```python
from build123d import *

# Parameters (mm, degrees)
SKETCH1_R           = 60.625
SKETCH1_R_2         = 45
BOSS_EXTRUDE1_DEPTH = 4
SKETCH2_R           = 49
SKETCH2_R_2         = 45
BOSS_EXTRUDE2_DEPTH = 52
SKETCH3_W           = 8
SKETCH3_H           = 38
SKETCH3_W_2         = 15
SKETCH3_H_2         = 8
BOSS_EXTRUDE3_DEPTH = 13
SKETCH4_W           = 10
SKETCH4_H           = 24
CUT_EXTRUDE1_DEPTH  = 8
SKETCH5_R           = 5
CUT_EXTRUDE2_DEPTH  = 110.441337026
SKETCH6_R           = 1.3
CUT_EXTRUDE3_DEPTH  = 7.2
BOSS_EXTRUDE4_DEPTH = 4
SKETCH8_R           = 1.5
CUT_EXTRUDE4_DEPTH  = 103.404986506
FILLET1_R           = 1


with BuildPart() as part:
    # Sketch1 → Boss-Extrude1 (new body)
    with BuildSketch(Plane(origin=(0, 0, 0), x_dir=(1, 0, 0), z_dir=(0, 1, 0))):
        with Locations(Location((0, 0, 0), (0, 0, 270))):
            Circle(SKETCH1_R)
        with Locations(Location((0, 0, 0), (0, 0, 270))):
            Circle(SKETCH1_R_2, mode=Mode.SUBTRACT)
    extrude(amount=BOSS_EXTRUDE1_DEPTH)

    # Sketch2 → Boss-Extrude2 (add)
    with BuildSketch(Plane(origin=(0, 4, 0), x_dir=(1, 0, 0), z_dir=(0, 1, 0))):
        with Locations(Location((0, 0, 0), (0, 0, 90))):
            Circle(SKETCH2_R)
        with Locations(Location((0, 0, 0), (0, 0, 270))):
            Circle(SKETCH2_R_2, mode=Mode.SUBTRACT)
    extrude(amount=BOSS_EXTRUDE2_DEPTH)

    # Sketch3 → Boss-Extrude3 (add, symmetric)
    with BuildSketch(Plane.XY):
        with Locations((15.25, 19)):
            Rectangle(SKETCH3_W, SKETCH3_H)
        with Locations((-39.25, 34)):
            Rectangle(SKETCH3_W_2, SKETCH3_H_2)
    extrude(amount=BOSS_EXTRUDE3_DEPTH, both=True)


with BuildPart() as boss_extrude3_piece_1:
    # of the separate pieces the step leaves, piece 1, a body of its own (boss_extrude3_pieces)
    add(part.part.solids().sort_by_distance((0, 0, 60.625))[0])

    # Sketch5 → Cut-Extrude2 (cut, through all)
    with BuildSketch(Plane.ZY.offset(-11.25)):
        with Locations((0, 14)):
            Circle(SKETCH5_R)
    extrude(amount=-CUT_EXTRUDE2_DEPTH, mode=Mode.SUBTRACT)


with BuildPart() as boss_extrude3_piece_2:
    # of the separate pieces the step leaves, piece 2, a body of its own (boss_extrude3_pieces)
    add(part.part.solids().sort_by_distance((11.25, 0, -13))[0])

    # Sketch4 → Cut-Extrude1 (cut)
    with BuildSketch(Plane.ZY.offset(-11.25)):
        with Locations((0, 17)):
            Rectangle(SKETCH4_W, SKETCH4_H)
    extrude(amount=-CUT_EXTRUDE1_DEPTH, mode=Mode.SUBTRACT)


with BuildPart() as cut_extrude3_tool:
    # Sketch6 → Cut-Extrude3 (new body)
    with BuildSketch(Plane(origin=(0, 38, 0), x_dir=(1, 0, 0), z_dir=(0, 1, 0))):
        with Locations(Location((-34.25, 5, 0), (0, 0, 270))):
            Circle(SKETCH6_R)
        with Locations(Location((-34.25, -5, 0), (0, 0, 270))):
            Circle(SKETCH6_R)
        with Locations(Location((13.75, 5, 0), (0, 0, 270))):
            Circle(SKETCH6_R)
        with Locations(Location((13.75, -5, 0), (0, 0, 270))):
            Circle(SKETCH6_R)
    extrude(amount=-CUT_EXTRUDE3_DEPTH)


with BuildPart() as boss_extrude3_piece_1_1:
    add(boss_extrude3_piece_1.part)

    # Cut-Extrude3: cut by cut_extrude3_tool
    add(cut_extrude3_tool.part, mode=Mode.SUBTRACT)



with BuildPart() as boss_extrude3_piece_2_1:
    add(boss_extrude3_piece_2.part)

    # Cut-Extrude3: cut by cut_extrude3_tool
    add(cut_extrude3_tool.part, mode=Mode.SUBTRACT)


with BuildPart() as boss_extrude3_piece_1_2:
    add(boss_extrude3_piece_1_1.part)

    add(boss_extrude3_piece_2_1.part)  # Boss-Extrude4 merges Boss-Extrude3 piece 2
    # Sketch7 → Boss-Extrude4 (add)
    with BuildSketch(Plane.XZ):
        with BuildLine():
            Line((11.25, -13), (25.249838503, -37.248431585))
            ThreePointArc((25.249838503, -37.248431585), (45, 0), (25.249838503, 37.248431585))
            Line((25.249838503, 37.248431585), (11.25, 13))
            Line((11.25, 13), (19.25, 13))
            Line((19.25, 13), (19.25, -13))
            Line((19.25, -13), (11.25, -13))
        make_face()
        with BuildLine():
            ThreePointArc((27.361802413, -24.906460381), (37, 0), (27.361802413, 24.906460381))
            Line((27.361802413, 24.906460381), (24.25, 19.516660498))
            Line((24.25, 19.516660498), (24.25, -19.516660498))
            Line((24.25, -19.516660498), (27.361802413, -24.906460381))
        make_face(mode=Mode.SUBTRACT)
    extrude(amount=-BOSS_EXTRUDE4_DEPTH)

    # Sketch8 → Cut-Extrude4 (cut, through all)
    with BuildSketch(Plane.XZ):
        with Locations(Location((54.5, 0, 0), (0, 0, 270))):
            Circle(SKETCH8_R)
        with Locations(Location((0, -54.5, 0), (0, 0, 270))):
            Circle(SKETCH8_R)
        with Locations(Location((-54.5, 0, 0), (0, 0, 270))):
            Circle(SKETCH8_R)
        with Locations(Location((0, 54.5, 0), (0, 0, 270))):
            Circle(SKETCH8_R)
    extrude(amount=-CUT_EXTRUDE4_DEPTH, mode=Mode.SUBTRACT)

    # Fillet1
    fillet1_edges = [boss_extrude3_piece_1_2.edges().sort_by_distance(p)[0] for p in [
        (0, 4, -60.625),
        (0, 4, 49),
    ]]
    fillet(fillet1_edges, radius=FILLET1_R)


solid = boss_extrude3_piece_1_2.part
```
Read the model definition and answer for the solid it produces. Units are mm, in the model's axes. A direction names the side the tool comes from. Coordinates: 2 decimals unless noted, no trailing zeros. Write each loop counter-clockwise with the first axis right and the second up, starting at its lowest first coordinate (ties: lowest second). Pieces come first, ordered by that corner, then holes. Notation, with made-up numbers: (74.25, -23.75) - (105.25, -23.75) arc R21 cw to (105.25, -7.75) - close; hole circle Ø2 at (27.25, 54.25). An arc over 180 degrees is marked (long way). Answer as a JSON object with one key per item and string values. Group by question number.
1. A cutting plane is placed at D-D (y = 40). Determine the outline of the cut face in (x, z), plus the area to 3 significant figures.
2. Consider L1, parallel to X at y = 31, z = -0.5; L2, parallel to Z at x = -34, y = 33; L3, parallel to X at y = 40, z = 0. Determine where each line is inside the solid, lowest interval first. Write a range as [from, to].
3. Which of the six approach directions +Z, -Z, +X, -X, +Y, -Y give full straight-line access (tool end or side, diameter ignored) to faces 1 (the flat face through (15, 21, -13)), 2 (the flat face through (11.25, 19, -6)), 3 (the flat face through (15, 17, 5)), 4 (the cylindrical face through (46.831, 18.957, -0.651))?
4. A cutting plane is placed at C-C (y = 10.5). Determine the outline of the cut face in (x, z).
5. Each of these flat-tipped pins is pushed along its axis until it touches: P1, Ø5, axis at x = 31, y = 40.5, coming from the +Z side; P2, Ø3, axis at y = 12, z = 29, coming from the -X side; P3, Ø2.5, axis at y = 34, z = 6, coming from the +X side. Where does it stop, or does it pass through?
6. A cutting plane is placed at B-B (z = 0). Give the number of separate pieces and of enclosed holes in the cut face, plus the area to 3 significant figures.
7. A cutting plane is placed at A-A (y = 22.5). Determine the outline of the cut face in (x, z).
8. The mould has two halves that part along Z. Classify faces 5 (the flat face through (-38, 38, 0)), 6 (the flat face through (15, 21, 13)), 7 (the cylindrical face through (-36.9, 1.5, -48.1)), 8 (the flat face through (-48.3, 4, -13.5)): +Z half, -Z half, draft (parallel to the pull), parting line (faces both ways), or undercut.
Worked out:
{
 "1": {"outline": "circle Ø98 at (0, 0); hole circle Ø90 at (0, 0)", "area": "1,180 mm²"},
 "2": {"L1": "x = [-49, -31.75], [11.25, 19.25], [45, 49]", "L2": "z = [-35.28, -29.48], [-13, -6.28], [-3.72, 3.72], [6.28, 13], [29.48, 35.28]", "L3": "x = [-49, -45], [45, 49]"},
 "3": {"face 1": "+Y", "face 2": "+Y, -Y", "face 3": "none", "face 4": "+X"},
 "4": {"outline": "(11.25, -13) - (19.25, -13) - (19.25, -5) - (11.25, -5) - close; (11.25, 5) - (19.25, 5) - (19.25, 13) - (11.25, 13) - close; (44.86, -3.57) arc R45 cw (long way) to (44.86, 3.57) - (48.87, 3.57) arc R49 ccw (long way) to (48.87, -3.57) - close"},
 "5": {"P1": "stops at z = 39.86", "P2": "stops at x = -40.56", "P3": "stops at x = 48.77"},
 "6": {"separate pieces": "7", "enclosed holes": "0", "area": "747 mm²"},
 "7": {"outline": "circle Ø98 at (0, 0); (11.25, -13) - (19.25, -13) - (19.25, -5) - (11.25, -5) - close; (11.25, 5) - (19.25, 5) - (19.25, 13) - (11.25, 13) - close; hole circle Ø90 at (0, 0)"},
 "8": {"face 5": "undercut", "face 6": "undercut", "face 7": "parting line", "face 8": "draft"}
}
